from build123d import *

# Parameters (mm, degrees)
SKETCH1_R           = 1.25
BOSS_EXTRUDE1_DEPTH = 3.175


with BuildPart() as part:
    # Sketch1 → Boss-Extrude1 (new body)
    with BuildSketch(Plane(origin=(0, 0, 0), x_dir=(1, 0, 0), z_dir=(0, 1, 0))):
        Polygon((0, 0), (10.675, 0), (21.35, 0), (21.35, 20), (21.35, 30), (0, 30), align=None)
        with BuildLine():
            ThreePointArc((12.175, 10), (11.735660172, 8.939339828), (10.675, 8.5))
            ThreePointArc((10.675, 8.5), (9.175, 10), (10.675, 11.5))
            ThreePointArc((10.675, 11.5), (11.735660172, 11.060660172), (12.175, 10))
        make_face(mode=Mode.SUBTRACT)
        with BuildLine():
            ThreePointArc((12.175, 20), (11.735660172, 18.939339828), (10.675, 18.5))
            ThreePointArc((10.675, 18.5), (9.614339828, 21.060660172), (12.175, 20))
        make_face(mode=Mode.SUBTRACT)
        with Locations(Location((17.35, 25, 0), (0, 0, 270))):
            Circle(SKETCH1_R, mode=Mode.SUBTRACT)
    extrude(amount=BOSS_EXTRUDE1_DEPTH)


solid = part.part
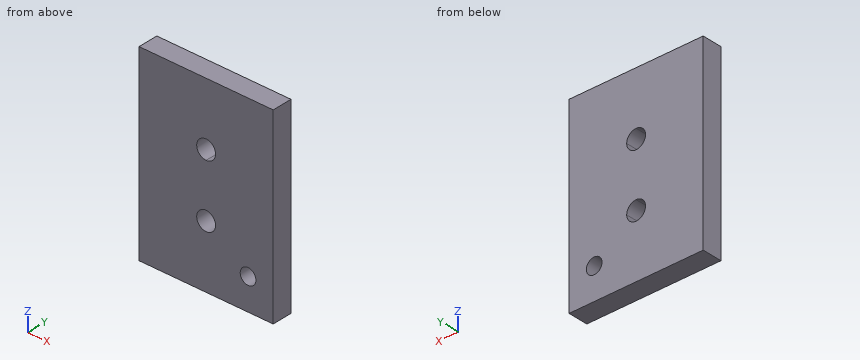
Design review of the part built by this model. Coordinates are the model's own, in mm. Coordinates: 2 decimals unless noted, no trailing zeros. Write each loop counter-clockwise with the first axis right and the second up, starting at its lowest first coordinate (ties: lowest second). Pieces come first, ordered by that corner, then holes. Notation, with made-up numbers: (-16.5, 67.5) - (6.5, 67.5) arc R36 cw to (6.5, 103.5) - close; hole circle Ø10 at (38, -21.5). An arc over 180 degrees is marked (long way). One line per item, written item: value.
1) Add section B-B (y = 0.7). State the section outline as (x, z) points (3 decimals), plus the area to 3 significant figures.
Answer sheet:
outline: (0, -30) - (21.35, -30) - (21.35, 0) - (0, 0) - close; hole circle Ø3 at (10.675, -20); hole circle Ø3 at (10.675, -10); hole circle Ø2.5 at (17.35, -25)
area: 621 mm2
2) Insertion check: pin 1 (2 mm diameter, centred on x = 17.35, z = -25, fed in from +Y). The pin has a flat end and moves straight along its axis. Give the tip position at first contact, or say it passes through.
Answer sheet:
pin 1: passes through
3) Add section C-C (z = -25). State the section outline as (x, y) points (3 decimals), plus the area to 3 significant figures.
Answer sheet:
outline: (0, 0) - (16.1, 0) - (16.1, 3.175) - (0, 3.175) - close; (18.6, 0) - (21.35, 0) - (21.35, 3.175) - (18.6, 3.175) - close
area: 59.8 mm2
4) Add section A-A (x = 17.35). State the section outline as (y, z) points (3 decimals).
Answer sheet:
outline: (0, -30) - (3.175, -30) - (3.175, -26.25) - (0, -26.25) - close; (0, -23.75) - (3.175, -23.75) - (3.175, 0) - (0, 0) - close
5) Add section D-D (x = 11.25). State the section outline as (y, z) points (3 decimals), plus the area to 3 significant figures.
Answer sheet:
outline: (0, -30) - (3.175, -30) - (3.175, -21.385) - (0, -21.385) - close; (0, -18.615) - (3.175, -18.615) - (3.175, -11.385) - (0, -11.385) - close; (0, -8.615) - (3.175, -8.615) - (3.175, 0) - (0, 0) - close
area: 77.7 mm2
6) To check wall thickness, follow probe 1 along X at (y, z) = (2.3, -25); probe 2 along X at (y, z) = (1.95, -20) (3 decimals); probe 3 along Z at (x, y) = (12, 0.25). State the ranges of each line that lie inside material, in increasing order.
Answer sheet:
probe 1: x = 0 to 16.1, 18.6 to 21.35
probe 2: x = 0 to 9.175, 12.175 to 21.35
probe 3: z = -30 to -20.7, -19.3 to -10.7, -9.3 to 0
